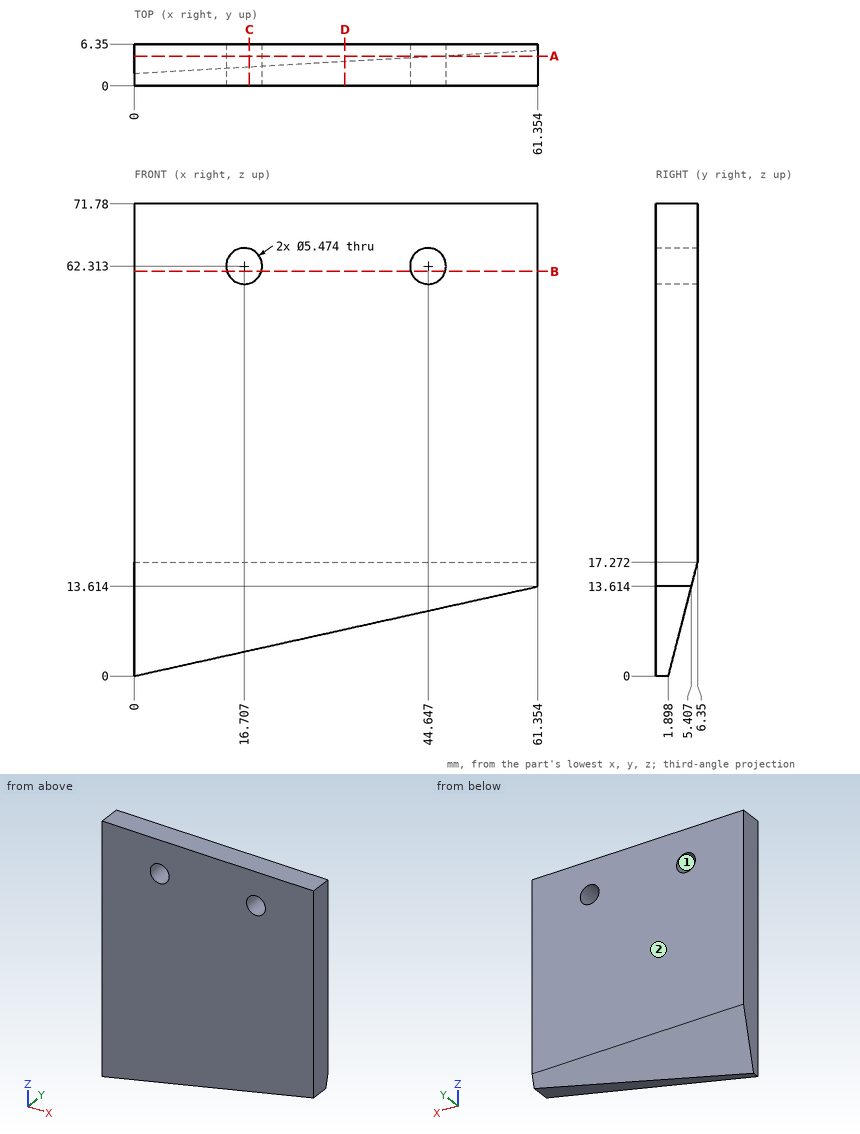
The drawing under review shows one solid part. Ordinate dimensions are in mm from its lowest x, y, z. Coordinates: 2 decimals unless noted, no trailing zeros. Loops run counter-clockwise (first coordinate to the right, second up) from the corner with the lowest first, then second, coordinate; pieces in that order, holes last.
Item 1: Add section C-C (x = 17.5). Write out the cut boundary in (y, z).
Completed:
outline: (0, 3.88) - (2.9, 3.88) - (6.35, 17.27) - (6.35, 59.69) - (0, 59.69) - close; (0, 64.93) - (6.35, 64.93) - (6.35, 71.78) - (0, 71.78) - close
Item 2: Add section D-D (x = 32). Write out the cut boundary in (y, z).
Completed:
outline: (0, 7.1) - (3.73, 7.1) - (6.35, 17.27) - (6.35, 71.78) - (0, 71.78) - close
Item 3: Draft analysis for pull direction X (two halves, no side actions). For the marked faces 1 and 2, state which applies: pulls with the +X half, pulls with the -X half, needs draft (parallel to the pull), parting line crosses it, or undercut.
Completed:
face 1: undercut
face 2: needs draft
Item 4: Wall thickness on L1, parallel to X at y = 6.25, z = 63 (1 decimal); L2, parallel to Z at x = 17, y = 2.75; L3, parallel to Z at x = 47, y = 4 (1 decimal): over which ranges is each line inside the solid? List them lowest first.
Completed:
L1: x = 0 to 14.1, 19.4 to 42, 47.3 to 61.4
L2: z = 3.77 to 59.59, 65.03 to 71.78
L3: z = 10.4 to 60.9, 63.7 to 71.8
Item 5: Add section A-A (y = 4.5). Write out the cut boundary in (x, z) (1 decimal), and give its area (3 significant figures).
Completed:
outline: (0, 10.1) - (45.5, 10.1) - (61.4, 13.6) - (61.4, 71.8) - (0, 71.8) - close; hole circle Ø5.5 at (16.7, 62.3); hole circle Ø5.5 at (44.6, 62.3)
area: 3,710 mm2
Item 6: Add section B-B (z = 61.5). Write out the cut boundary in (x, y).
Completed:
outline: (0, 0) - (14.09, 0) - (14.09, 6.35) - (0, 6.35) - close; (19.32, 0) - (42.03, 0) - (42.03, 6.35) - (19.32, 6.35) - close; (47.26, 0) - (61.35, 0) - (61.35, 6.35) - (47.26, 6.35) - close
